Read the model definition and answer for the solid it produces. Units are mm, in the model's axes. A direction names the side the tool comes from. Coordinates: 2 decimals unless noted, no trailing zeros. Loops run counter-clockwise (first coordinate to the right, second up) from the corner with the lowest first, then second, coordinate; pieces in that order, holes last. Notation, with made-up numbers: M -11,21.25 L 32,21.25 A29 cw 32,60.25 Z; hole C -20,55.5 d10. An arc over 180 degrees is marked long. Put each result on its own line as item: value.
from build123d import *

# Parameters (mm, degrees)
BOSS_EXTRUDE1_DEPTH = 2
BOSS_EXTRUDE2_DEPTH = 2
SKETCH4_W           = 60.5
SKETCH4_H           = 8
BOSS_EXTRUDE3_DEPTH = 2
SKETCH5_R           = 1
CUT_EXTRUDE1_DEPTH  = 1
CUT_EXTRUDE2_DEPTH  = 1


with BuildPart() as part:
    # Sketch1 → Boss-Extrude1 (new body)
    with BuildSketch(Plane.XY):
        with BuildLine():
            Line((23.840057871, 8), (-24.840057871, 8))
            add(Edge.make_bspline(
                [(-24.840057871, 8), (-29.579374102, 7.859454073), (-32.25, 4.777235297)],
                knots=[0, 0, 0, 1, 1, 1], degree=2))
            Line((-32.25, 4.777235297), (-32.25, -8))
            Line((-32.25, -8), (31.25, -8))
            Line((31.25, -8), (31.25, 4.777235297))
            add(Edge.make_bspline(
                [(23.840057871, 8), (28.579374102, 7.859454073), (31.25, 4.777235297)],
                knots=[0, 0, 0, 1, 1, 1], degree=2))
        make_face()
    extrude(amount=BOSS_EXTRUDE1_DEPTH)

    # Sketch2 → Boss-Extrude2 (add)
    with BuildSketch(Plane.XY.offset(2)):
        with BuildLine():
            Line((-32.25, -8), (31.25, -8))
            Line((31.25, -8), (31.250000012, 4.777235284))
            add(Edge.make_bspline(
                [(31.250000012, 4.777235284), (28.579374112, 7.859454073), (23.840057871, 8)],
                knots=[0, 0, 0, 1, 1, 1], degree=2))
            Line((23.840057871, 8), (-24.84005786, 8))
            add(Edge.make_bspline(
                [(-24.84005786, 8), (-29.579374099, 7.859454077), (-32.25, 4.777235297)],
                knots=[0, 0, 0, 1, 1, 1], degree=2))
            Line((-32.25, 4.777235297), (-32.25, -8))
        make_face()
        with BuildLine():
            Line((-31.25, -7), (30.25, -7))
            Line((30.25, -7), (30.250000006, 4.392275401))
            add(Edge.make_bspline(
                [(30.250000006, 4.392275401), (29.838936293, 4.827054032), (29.388289272, 5.208885934), (28.405623687, 5.863706962), (27.867648486, 6.137833076), (26.761664402, 6.561008933), (26.189843053, 6.714315907), (25.015344092, 6.925422761), (24.421635521, 6.981682834), (23.824977184, 7)],
                knots=[0, 0, 0, 0, 0.25, 0.25, 0.5, 0.5, 0.75, 0.75, 1, 1, 1, 1], degree=3))
            Line((23.824977184, 7), (-24.824977186, 7))
            add(Edge.make_bspline(
                [(-24.824977186, 7), (-25.421773324, 6.981678604), (-26.010765986, 6.925523135), (-27.169262236, 6.718722121), (-27.738796388, 6.568224766), (-28.574197272, 6.250843034), (-28.850434321, 6.12895654), (-29.381068271, 5.858126444), (-29.893359619, 5.559169961), (-30.368382987, 5.203067082), (-30.824570304, 4.818081166), (-31.043507271, 4.610681029), (-31.25, 4.392275407)],
                knots=[0, 0, 0, 0, 0.25, 0.25, 0.5, 0.5, 0.625, 0.625, 0.75, 0.875, 0.875, 1, 1, 1, 1], degree=3))
            Line((-31.25, 4.392275407), (-31.25, -7))
        make_face(mode=Mode.SUBTRACT)
    extrude(amount=BOSS_EXTRUDE2_DEPTH)

    # Sketch4 → Boss-Extrude3 (add)
    with BuildSketch(Plane.XY.offset(4)):
        with BuildLine():
            Line((-32.25, -8), (31.25, -8))
            Line((31.25, -8), (31.250000012, 4.777235284))
            add(Edge.make_bspline(
                [(31.250000012, 4.777235284), (28.579374112, 7.859454073), (23.840057871, 8)],
                knots=[0, 0, 0, 1, 1, 1], degree=2))
            Line((23.840057871, 8), (-24.84005786, 8))
            add(Edge.make_bspline(
                [(-24.84005786, 8), (-29.579374099, 7.859454077), (-32.25, 4.777235297)],
                knots=[0, 0, 0, 1, 1, 1], degree=2))
            Line((-32.25, 4.777235297), (-32.25, -8))
        make_face()
        Rectangle(SKETCH4_W, SKETCH4_H, mode=Mode.SUBTRACT)
    extrude(amount=BOSS_EXTRUDE3_DEPTH)

    # Sketch5 → Cut-Extrude1 (cut)
    with BuildSketch(Plane.XY.offset(2)):
        with Locations((-26.25, 0)):
            Circle(SKETCH5_R)
    extrude(amount=-CUT_EXTRUDE1_DEPTH, mode=Mode.SUBTRACT)

    # Sketch6 → Cut-Extrude2 (cut)
    with BuildSketch(Plane(origin=(0, 0, 0), x_dir=(-1, 0, 0), z_dir=(0, 0, -1))):
        with BuildLine():
            Line((24.840057871, 8), (31.25, 8))
            Line((31.25, 8), (32.25, 4.777235297))
            add(Edge.make_bspline(
                [(24.840057871, 8), (29.579374102, 7.859454073), (32.25, 4.777235297)],
                knots=[0, 0, 0, 1, 1, 1], degree=2))
        make_face()
    cut_extrude2 = extrude(amount=-CUT_EXTRUDE2_DEPTH, mode=Mode.SUBTRACT)

    # Mirror1: Cut-Extrude2 across plane
    add(cut_extrude2.mirror(Plane(origin=(0, 0, 0), x_dir=(0, 0, 1), z_dir=(1, 0, 0))), mode=Mode.SUBTRACT)


solid = part.part
1) Determine the mould class of faces 4 (the cylindrical face through (-27.25, 0.04, 1.51)), 5 (the flat face through (-32.25, -2, 3)), 6 (the flat face through (-1, -8, 3)) for opening direction X: released by +X, released by -X, zero draft, split by the parting line, or undercut.
Answer list:
face 4: undercut
face 5: released by -X
face 6: zero draft
2) Given pin 1 Ø1.6 at (x, y) = (-26.5, -0.5) entering from +Z; pin 2 Ø2.5 at (x, y) = (-26.25, 0) entering from -Z, each flat-ended and moving along its own axis, determine where each tip first touches the part or whether it passes through.
Answer list:
pin 1: stops at z = 2
pin 2: stops at z = 0
3) Find section B-B, the plane y = 0. Write down the section's boundary in (x, z), plus the area to 3 significant figures.
Answer list:
outline: M -32.25,0 L 31.25,0 L 31.25,6 L 30.25,6 L 30.25,2 L -25.25,2 L -25.25,1 L -27.25,1 L -27.25,2 L -31.25,2 L -31.25,4 L -30.25,4 L -30.25,6 L -32.25,6 Z
area: 135 mm^2
4) Straight lines are drawn through the part: line 1 (X direction, y = 2.75, z = 3.5); line 2 (Y direction, x = -13.5, z = 2.25). For each, find the intervals that lie inside material, in ascending order. Write a range as [from, to].
Answer list:
line 1: x = [-32.25, -31.25], [30.25, 31.25]
line 2: y = [-8, -7], [7, 8]
5) Which of the six approach directions +Z, -Z, +X, -X, +Y, -Y give full straight-line access (tool end or side, diameter ignored) to faces 1 (the flat face through (-31.25, -1, 3)), 2 (the flat face through (-1, -5, 6)), 3 (the flat face through (0, 4, 5))?
Answer list:
face 1: none
face 2: +Z, +X, -X, +Y, -Y
face 3: +Z
6) Find section A-A, the plane x = 1. Write down the section's boundary in (y, z), plus the area to 3 significant figures.
Answer list:
outline: M -8,0 L 8,0 L 8,6 L 4,6 L 4,4 L 7,4 L 7,2 L -7,2 L -7,4 L -4,4 L -4,6 L -8,6 Z
area: 52.0 mm^2
